Build history of the part. All positions in model axes, mm. Face numbers are marked on the shaded views. A direction names the side the tool comes from. Give positions to 0.01 mm unless a question says otherwise; leave off trailing zeros. Loops run counter-clockwise (first coordinate to the right, second up) from the corner with the lowest first, then second, coordinate; pieces in that order, holes last. Notation, with made-up numbers: (56, 77) -> (85, 77) arc R21 ccw to (85, 95) -> close; hole circle Ø8 at (80, -3). An arc over 180 degrees is marked (long way). One line per question, with ' | ' between items. Start each with the question number.
(1) Slice it at B-B, the plane z = 20. Write the cut outline in (x, y), then the cut area to 3 significant figures.
(2) Slice it at D-D, the plane x = -11. Write the cut outline in (y, z), then the cut area to 3 significant figures.
(3) Drill centre lines: L1, parallel to X at y = 5, z = 10; L2, parallel to Y at x = 27, z = 10.75; L3, parallel to Z at x = -8.5, y = 34. Where is each one in solid material? Low to high. Write a range as from..to.
(4) 3-axis set-ups, long thin cutter, end or side, ignore diameter. For the marked faces 4 and 5: which of +Z, -Z, +X, -X, +Y, -Y reach the whole face in a straight line?
(5) Slice it at C-C, the plane y = 1. Write the cut outline in (x, z).
(6) Mould opens along Y. For the marked faces 1, 2 and 3 say: pulls with the +Y half, pulls with the -Y half, needs draft (parallel to the pull), parting line crosses it, or undercut.
(7) Flat gauge pins, fed straight in: pin 1 Ø0.7 at (x, y) = (6.5, -30) entering from +Z; pin 2 Ø1 at (x, y) = (33, -18) entering from +Z. Where does each tip first touch, or does it go through?
(8) Slice it at A-A, the plane x = 33. Write the cut outline in (y, z).
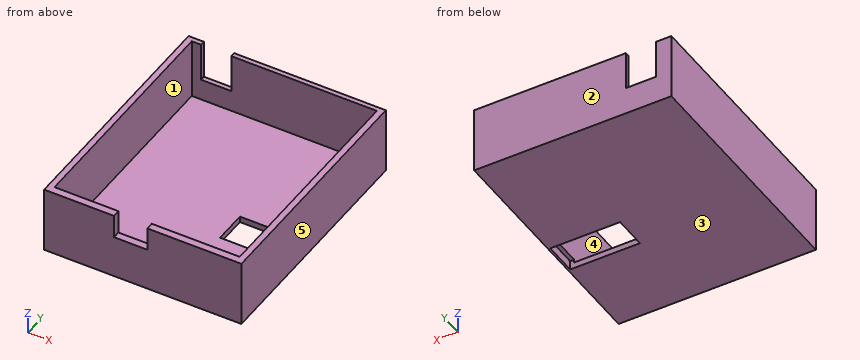
```python
from build123d import *

# Parameters (mm, degrees)
SCHIZZO1_W                   = 65
SCHIZZO1_H                   = 80
ESTRUSIONE_ESTRUSIONE1_DEPTH = 22
SCHIZZO2_W                   = 61
SCHIZZO2_H                   = 76
TAGLIO_ESTRUSIONE1_DEPTH     = 20
SCHIZZO4_W                   = 11
SCHIZZO4_H                   = 8.5
TAGLIO_ESTRUSIONE2_DEPTH     = 3
SCHIZZO5_W                   = 23
SCHIZZO5_H                   = 11
TAGLIO_ESTRUSIONE3_DEPTH     = 3
SCHIZZO6_W                   = 10
SCHIZZO6_H                   = 14
TAGLIO_ESTRUSIONE4_DEPTH     = 3


with BuildPart() as part:
    # Schizzo1 → Estrusione-Estrusione1 (new body)
    with BuildSketch(Plane.XY):
        with Locations((8.270457538, 8.882113821)):
            Rectangle(SCHIZZO1_W, SCHIZZO1_H)
    extrude(amount=ESTRUSIONE_ESTRUSIONE1_DEPTH)

    # Schizzo2 → Taglio-Estrusione1 (cut)
    with BuildSketch(Plane.XY.offset(22)):
        with Locations((8.235197237, 9.324988178)):
            Rectangle(SCHIZZO2_W, SCHIZZO2_H)
    extrude(amount=-TAGLIO_ESTRUSIONE1_DEPTH, mode=Mode.SUBTRACT)

    # Schizzo4 → Taglio-Estrusione2 (cut)
    with BuildSketch(Plane.XZ.offset(31.117886179)):
        with Locations((4.269357769, 18.454892341)):
            Rectangle(SCHIZZO4_W, SCHIZZO4_H)
    extrude(amount=-TAGLIO_ESTRUSIONE2_DEPTH, mode=Mode.SUBTRACT)

    # Schizzo5 → Taglio-Estrusione3 (cut)
    with BuildSketch(Plane(origin=(0, 0, 0), x_dir=(-1, 0, 0), z_dir=(0, 0, -1))):
        with Locations((-28.573968875, 2.379418808)):
            Rectangle(SCHIZZO5_W, SCHIZZO5_H)
    extrude(amount=-TAGLIO_ESTRUSIONE3_DEPTH, mode=Mode.SUBTRACT)

    # Schizzo6 → Taglio-Estrusione4 (cut)
    with BuildSketch(Plane(origin=(0, 48.882113821, 0), x_dir=(1, 0, 0), z_dir=(0, 1, 0))):
        with Locations((-14.227965798, -16.217758031)):
            Rectangle(SCHIZZO6_W, SCHIZZO6_H)
    extrude(amount=-TAGLIO_ESTRUSIONE4_DEPTH, mode=Mode.SUBTRACT)


solid = part.part
```
Final values:
1) outline: (-24.23, -31.12) -> (-1.23, -31.12) -> (-1.23, -28.68) -> (-22.26, -28.68) -> (-22.26, 47.32) -> (-19.23, 47.32) -> (-19.23, 48.88) -> (-24.23, 48.88) -> close; (-9.23, 47.32) -> (38.74, 47.32) -> (38.74, -28.68) -> (9.77, -28.68) -> (9.77, -31.12) -> (40.77, -31.12) -> (40.77, 48.88) -> (-9.23, 48.88) -> close | area: 522 mm2
2) outline: (-31.12, 0) -> (48.88, 0) -> (48.88, 9.22) -> (47.32, 9.22) -> (47.32, 2) -> (-28.68, 2) -> (-28.68, 22) -> (-31.12, 22) -> close | area: 220 mm2
3) L1: -24.23..-22.26, 38.74..40.77 | L2: -31.12..-28.68, 47.32..48.88 | L3: 0..2
4) face 4: +Z | face 5: +Z, -Z, +X, +Y, -Y
5) outline: (-24.23, 0) -> (17.07, 0) -> (17.07, 2) -> (-22.26, 2) -> (-22.26, 22) -> (-24.23, 22) -> close; (38.74, 3) -> (40.07, 3) -> (40.07, 0) -> (40.77, 0) -> (40.77, 22) -> (38.74, 22) -> close
6) face 1: undercut | face 2: pulls with the +Y half | face 3: needs draft
7) pin 1: z = 14.2 | pin 2: z = 2
8) outline: (-31.12, 0) -> (-3.12, 0) -> (-3.12, 2) -> (-28.68, 2) -> (-28.68, 22) -> (-31.12, 22) -> close; (7.88, 0) -> (48.88, 0) -> (48.88, 22) -> (47.32, 22) -> (47.32, 2) -> (7.88, 2) -> close
